Design review of the part built by this model. Coordinates are the model's own, in mm. Face numbers are marked on the shaded views. A direction names the side the tool comes from. Coordinates: 2 decimals unless noted, no trailing zeros. Write each loop counter-clockwise with the first axis right and the second up, starting at its lowest first coordinate (ties: lowest second). Pieces come first, ordered by that corner, then holes. Notation, with made-up numbers: (-37, -24) - (9, -24) arc R17 ccw to (9, 9) - close; hole circle Ø7 at (7, -36). An arc over 180 degrees is marked (long way). Use a Markdown table: item, result.
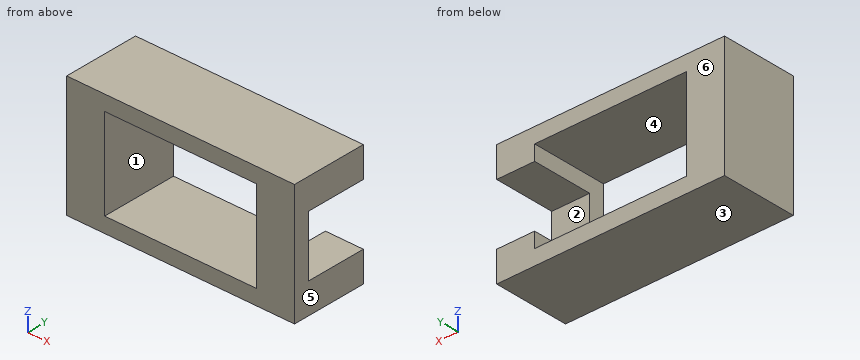
from build123d import *

# Parameters (mm, degrees)
CUT_EXTRUDE3_DEPTH           = 60
CUT_EXTRUDE5_DEPTH           = 2
CUT_EXTRUDE5_DEPTH_BACK      = 30
SKETCH9_R                    = 38
SKETCH9_R_2                  = 23
SKETCH19_W                   = 12
SKETCH19_H                   = 36.5
CUT_REVOLVE2_ANGLE           = 65
CUT_REVOLVE2_OTHER_WAY_ANGLE = 65
SKETCH21_W                   = 3.25
SKETCH21_H                   = 4
BOSS_EXTRUDE3_DEPTH          = 1.35
CIRPATTERN1_COUNT            = 5
CUT_EXTRUDE9_START           = -5
CUT_EXTRUDE9_DEPTH           = 5
SKETCH23_R                   = 10.5
CUT_EXTRUDE10_DEPTH          = 10
SKETCH24_W                   = 15
SKETCH24_H                   = 8
BOSS_EXTRUDE4_DEPTH          = 8
SKETCH26_W                   = 10
SKETCH26_H                   = 6
CUT_EXTRUDE11_DEPTH          = 10
SKETCH27_W                   = 4
SKETCH27_H                   = 5
CUT_EXTRUDE12_DEPTH          = 5
CUT_EXTRUDE14_DEPTH          = 2
CUT_EXTRUDE14_DEPTH_BACK     = 30
SKETCH29_R                   = 1
CUT_EXTRUDE15_DEPTH          = 15
FILLET1_R                    = 6
FILLET2_R                    = 8
INTERSECT1_OUTLINE_W         = 15
INTERSECT1_OUTLINE_H         = 8
INTERSECT1_OUTLINE_W_2       = 10
INTERSECT1_OUTLINE_H_2       = 6
INTERSECT1_DEPTH             = 63.427876097
INTERSECT1_START             = 13
INTERSECT1_2_OUTLINE_W       = 15
INTERSECT1_2_OUTLINE_H       = 8
INTERSECT1_2_OUTLINE_W_2     = 10
INTERSECT1_2_OUTLINE_H_2     = 6
INTERSECT1_2_DEPTH           = 12.427876097
INTERSECT1_START_2           = 55.427876097
INTERSECT1_3_OUTLINE_W       = 15
INTERSECT1_3_OUTLINE_H       = 8
INTERSECT1_3_OUTLINE_W_2     = 10
INTERSECT1_3_OUTLINE_H_2     = 6
INTERSECT1_3_DEPTH           = 3


# Read off the part's stored shape, not the designer's step: Cut-Extrude9, Intersect1
with BuildPart() as part:
    # Sketch1 → Revolve1 (revolve)
    with BuildSketch(Plane.XY, mode=Mode.PRIVATE) as revolve1_sk:
        with BuildLine():
            Line((0, 63.427876097), (32, 63.427876097))
            ThreePointArc((32, 63.427876097), (37.656854249, 61.084730346), (40, 55.427876097))
            Line((40, 55.427876097), (40, 28.846818009))
            ThreePointArc((40, 28.846818009), (38.792081772, 24.082439968), (35.460140376, 20.469057744))
            Line((35.460140376, 20.469057744), (28.539859624, 15.958818353))
            ThreePointArc((28.539859624, 15.958818353), (25.207918228, 12.345436129), (24, 7.581058088))
            Line((24, 7.581058088), (24, 3.25))
            Line((24, 3.25), (24.35, 3))
            Line((24.35, 3), (24.35, 0))
            Line((24.35, 0), (22.5, 0))
            Line((22.5, 0), (22.5, 12.5))
            ThreePointArc((22.5, 12.5), (22.353553391, 12.853553391), (22, 13))
            Line((22, 13), (0, 13))
            Line((0, 13), (0, 63.427876097))
        make_face()
    revolve(revolve1_sk.sketch.rotate(Axis((0, 0, 0), (0, 1, 0)), 90), axis=Axis((0, 0, 0), (0, 1, 0)))

    # Sketch11 → Cut-Extrude3 (cut)
    with BuildSketch(Plane(origin=(0, 13, 0), x_dir=(-1, 0, 0), z_dir=(0, -1, 0))):
        with BuildLine():
            Line((-21, 0), (21, 0))
            ThreePointArc((21, 0), (0, 21), (-21, 0))
        make_face()
    extrude(amount=-CUT_EXTRUDE3_DEPTH, mode=Mode.SUBTRACT)

    # Sketch9 → Cut-Extrude5 (cut, two sides: drawn at the far end of the back side and taken through both)
    with BuildSketch(Plane(origin=(0, 55.427876097, 0), x_dir=(1, 0, 0), z_dir=(0, 1, 0)).offset(-CUT_EXTRUDE5_DEPTH_BACK)):
        with Locations(Location((0, 0, 0), (0, 0, 270))):
            Circle(SKETCH9_R)
        with Locations(Location((0, 0, 0), (0, 0, 270))):
            Circle(SKETCH9_R_2, mode=Mode.SUBTRACT)
    extrude(amount=CUT_EXTRUDE5_DEPTH + CUT_EXTRUDE5_DEPTH_BACK, mode=Mode.SUBTRACT)

    # Sketch19 → Cut-Revolve2 (revolve, cut)
    with BuildSketch(Plane(origin=(0, 0, 0), x_dir=(0, 0, -1), z_dir=(1, 0, 0))):
        with Locations((-41.064715832, 37.177876097)):
            Rectangle(SKETCH19_W, SKETCH19_H)
    revolve(axis=Axis((0, 0, 0), (0, 1, 0)), revolution_arc=CUT_REVOLVE2_ANGLE, mode=Mode.SUBTRACT)

    # Sketch19 → Cut-Revolve2 other way (revolve, cut)
    with BuildSketch(Plane(origin=(0, 0, 0), x_dir=(0, 0, -1), z_dir=(1, 0, 0))):
        with Locations((-41.064715832, 37.177876097)):
            Rectangle(SKETCH19_W, SKETCH19_H)
    revolve(axis=Axis((0, 0, 0), (0, -1, 0)), revolution_arc=CUT_REVOLVE2_OTHER_WAY_ANGLE, mode=Mode.SUBTRACT)

    # Sketch21 → Boss-Extrude3 (add)
    with BuildSketch(Plane(origin=(0, 0, 22.5), x_dir=(-1, 0, 0), z_dir=(0, 0, -1))):
        with Locations((0, 2)):
            Rectangle(SKETCH21_W, SKETCH21_H)
    boss_extrude3 = extrude(amount=BOSS_EXTRUDE3_DEPTH)

    # CirPattern1: Boss-Extrude3 ×5 about axis
    cirpattern1_axis = Axis((0, 0, 0), (0, 1, 0))
    for i in range(1, CIRPATTERN1_COUNT):
        add(boss_extrude3.rotate(cirpattern1_axis, i * 360 / CIRPATTERN1_COUNT))

    # Cut-Extrude9 outline → Cut-Extrude9 (cut)
    with BuildSketch(Plane(origin=(0, 63.427876097, 0), x_dir=(1, 0, 0), z_dir=(0, 1, 0)).offset(CUT_EXTRUDE9_START)):
        with BuildLine():
            ThreePointArc((40, 0), (0, 40), (-40, 0))
            Line((-40, 0), (-21, 0))
            ThreePointArc((-21, 0), (0, 21), (21, 0))
            Line((21, 0), (40, 0))
        make_face()
    extrude(amount=CUT_EXTRUDE9_DEPTH, mode=Mode.SUBTRACT)

    # Sketch23 → Cut-Extrude10 (cut)
    with BuildSketch(Plane(origin=(0, 0, -40), x_dir=(-1, 0, 0), z_dir=(0, 0, -1))):
        with Locations((0, 42.137876097)):
            Circle(SKETCH23_R)
    extrude(amount=-CUT_EXTRUDE10_DEPTH, mode=Mode.SUBTRACT)

    # Sketch24 → Boss-Extrude4 (add)
    with BuildSketch(Plane(origin=(0, 58.427876097, 0), x_dir=(1, 0, 0), z_dir=(0, 1, 0))):
        with Locations((0, 30)):
            Rectangle(SKETCH24_W, SKETCH24_H)
    extrude(amount=-BOSS_EXTRUDE4_DEPTH)

    # Sketch26 → Cut-Extrude11 (cut)
    with BuildSketch(Plane(origin=(0, 58.427876097, 0), x_dir=(1, 0, 0), z_dir=(0, 1, 0))):
        with Locations((0, 30)):
            Rectangle(SKETCH26_W, SKETCH26_H)
    extrude(amount=-CUT_EXTRUDE11_DEPTH, mode=Mode.SUBTRACT)

    # Sketch27 → Cut-Extrude12 (cut)
    with BuildSketch(Plane(origin=(7.5, 0, 0), x_dir=(0, 0, -1), z_dir=(1, 0, 0))):
        with Locations((30, 53.927876097)):
            Rectangle(SKETCH27_W, SKETCH27_H)
    extrude(amount=-CUT_EXTRUDE12_DEPTH, mode=Mode.SUBTRACT)

    # Sketch28 → Cut-Extrude14 (cut, two sides: drawn at the far end of the back side and taken through both)
    with BuildSketch(Plane(origin=(0, 55.427876097, 0), x_dir=(1, 0, 0), z_dir=(0, 1, 0)).offset(-CUT_EXTRUDE14_DEPTH_BACK)):
        with BuildLine():
            Line((-22.912878475, -2), (22.912878475, -2))
            ThreePointArc((22.912878475, -2), (0, -23), (-22.912878475, -2))
        make_face()
    extrude(amount=CUT_EXTRUDE14_DEPTH + CUT_EXTRUDE14_DEPTH_BACK, mode=Mode.SUBTRACT)

    # Sketch29 → Cut-Extrude15 (cut)
    with BuildSketch(Plane(origin=(0, 0, 0), x_dir=(-1, 0, 0), z_dir=(0, 0, -1))):
        with Locations((-30.416198487, 60.927876097)):
            Circle(SKETCH29_R)
        with Locations((30.416198487, 60.927876097)):
            Circle(SKETCH29_R)
        with Locations((0, 60.927876097)):
            Circle(SKETCH29_R)
    extrude(amount=-CUT_EXTRUDE15_DEPTH, mode=Mode.SUBTRACT)

    # Fillet1
    fillet1_edges = [part.edges().sort_by_distance(p)[0] for p in [
        (21, 35.713938048, 0),
        (-21, 35.713938048, 0),
    ]]
    fillet(fillet1_edges, radius=FILLET1_R)

    # Fillet2
    fillet2_edges = [part.edges().sort_by_distance(p)[0] for p in [
        (-22.912878475, 41.427876097, 2),
        (22.912878475, 41.427876097, 2),
    ]]
    fillet(fillet2_edges, radius=FILLET2_R)

    # Intersect1 outline → Intersect1 (cut)
    # profile 1 of 2: a face of its own
    with BuildSketch(Plane(origin=(0, 0, 0), x_dir=(1, 0, 0), z_dir=(0, 1, 0))):
        with BuildLine():
            Line((-37.080992435, -15), (-40.906642577, -15))
            Line((-40.906642577, -15), (-42, -15.355253362))
            Line((-42, -15.355253362), (-42, -42))
            Line((-42, -42), (42, -42))
            Line((42, -42), (42, -15.355253362))
            Line((42, -15.355253362), (40.906642577, -15))
            Line((40.906642577, -15), (37.080992435, -15))
            ThreePointArc((37.080992435, -15), (0, 40), (-37.080992435, -15))
        make_face()
        with BuildLine():
            ThreePointArc((19.246817919, 8.4), (18.767687244, 2.713664655), (13.747727085, 0))
            Line((13.747727085, 0), (-13.747727085, 0))
            ThreePointArc((-13.747727085, 0), (-18.767687244, 2.713664655), (-19.246817919, 8.4))
            ThreePointArc((-19.246817919, 8.4), (0, 21), (19.246817919, 8.4))
        make_face(mode=Mode.SUBTRACT)
        with Locations((0, 30)):
            Rectangle(INTERSECT1_OUTLINE_W, INTERSECT1_OUTLINE_H, mode=Mode.SUBTRACT)
    # profile 2 of 2: a face of its own
    with BuildSketch(Plane(origin=(0, 0, 0), x_dir=(1, 0, 0), z_dir=(0, 1, 0))):
        with Locations((0, 30)):
            Rectangle(INTERSECT1_OUTLINE_W_2, INTERSECT1_OUTLINE_H_2)
    extrude(amount=INTERSECT1_DEPTH, mode=Mode.SUBTRACT)

    # Intersect1 2 outline → Intersect1 2 (cut)
    with BuildSketch(Plane(origin=(0, 0, 0), x_dir=(1, 0, 0), z_dir=(0, 1, 0)).offset(INTERSECT1_START)):
        with Locations((0, 30)):
            Rectangle(INTERSECT1_2_OUTLINE_W, INTERSECT1_2_OUTLINE_H)
        with Locations((0, 30)):
            Rectangle(INTERSECT1_2_OUTLINE_W_2, INTERSECT1_2_OUTLINE_H_2, mode=Mode.SUBTRACT)
    extrude(amount=INTERSECT1_2_DEPTH, mode=Mode.SUBTRACT)

    # Intersect1 3 outline → Intersect1 3 (cut)
    with BuildSketch(Plane(origin=(0, 0, 0), x_dir=(1, 0, 0), z_dir=(0, 1, 0)).offset(INTERSECT1_START_2)):
        with Locations((0, 30)):
            Rectangle(INTERSECT1_3_OUTLINE_W, INTERSECT1_3_OUTLINE_H)
        with Locations((0, 30)):
            Rectangle(INTERSECT1_3_OUTLINE_W_2, INTERSECT1_3_OUTLINE_H_2, mode=Mode.SUBTRACT)
    extrude(amount=INTERSECT1_3_DEPTH, mode=Mode.SUBTRACT)


solid = part.part
(1) Take a section at B-B on z = -30. Write out the cut boundary in (x, y), and give its area (3 significant figures).
Determined:
| item | result |
|---|---|
| outline | (-7.5, 50.43) - (-5, 50.43) - (-5, 55.43) - (-7.5, 55.43) - close; (5, 50.43) - (7.5, 50.43) - (7.5, 51.43) - (5, 51.43) - close |
| area | 15.0 mm2 |
(2) Take a section at D-D on x = 6.75. Write out the cut boundary in (y, z), and give its area (3 significant figures).
Determined:
| item | result |
|---|---|
| outline | (50.43, -34) - (55.43, -34) - (55.43, -32) - (51.43, -32) - (51.43, -28) - (55.43, -28) - (55.43, -26) - (50.43, -26) - close |
| area | 24.0 mm2 |
(3) Take a section at A-A on x = 2.25. Write out the cut boundary in (y, z), and give its area (3 significant figures).
Determined:
| item | result |
|---|---|
| outline | (50.43, -34) - (55.43, -34) - (55.43, -33) - (50.43, -33) - close; (50.43, -27) - (55.43, -27) - (55.43, -26) - (50.43, -26) - close |
| area | 10.0 mm2 |
(4) For L1, parallel to X at y = 52.8, z = -32.75; L2, parallel to Z at x = -4, y = 51; L3, parallel to Z at x = 7.25, y = 54.7, list the stretches that pass through material, from the lowest coordinate up. Write a range as from..to.
Determined:
| item | result |
|---|---|
| L1 | -7.5..-5, 5..7.5 |
| L2 | -34..-33, -27..-26 |
| L3 | -34..-32, -28..-26 |
(5) Take a section at C-C on y = 54.9. Write out the cut boundary in (x, z).
Determined:
| item | result |
|---|---|
| outline | (-7.5, -34) - (7.5, -34) - (7.5, -32) - (5, -32) - (5, -33) - (-5, -33) - (-5, -27) - (5, -27) - (5, -28) - (7.5, -28) - (7.5, -26) - (-7.5, -26) - close |
(6) Draft analysis for pull direction X (two halves, no side actions). For the marked faces 4, 5 and 6, state which applies: +X half, -X half, draft (parallel to the pull), parting line (faces both ways), or undercut.
Determined:
| item | result |
|---|---|
| face 4 | undercut |
| face 5 | +X half |
| face 6 | draft |
(7) Machinability: for the marked faces 1, 2 and 3, which of the approach directions +Z, -Z, +X, -X, +Y, -Y give a long, thin tool a straight path to every point of the face, cutting with its end or side? Answer none if there is none.
Determined:
| item | result |
|---|---|
| face 1 | +Y, -Y |
| face 2 | +X, +Y |
| face 3 | -Z, +X, -X, +Y, -Y |
